Input: part model. Units: mm. Frame: model coordinates. Face numbers are marked on the shaded views. A direction names the side the tool comes from. Coordinates: 2 decimals unless noted, no trailing zeros. Order: outer loops, then holes, each group sorted by start corner. A loop starts at its lowest first (then second) coordinate and runs counter-clockwise, first axis right, second up. Notation, with made-up numbers: (35.25, 36) -> (43.25, 36) arc R14 cw to (43.25, 61) -> close; hole circle Ø2 at (86.5, -27). An arc over 180 degrees is marked (long way). One line per question, with ' | ' between items.
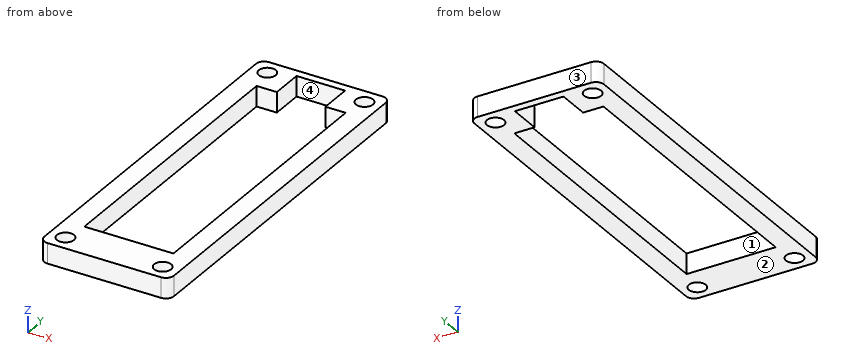
```python
from build123d import *

# Parameters (mm, degrees)
SKETCH_W      = 32
SKETCH_H      = 90
SKETCH_R      = 2.1
EXTRUDE_DEPTH = 5
FILLET_R      = 2


with BuildPart() as part:
    # Sketch → Extrude (new body)
    with BuildSketch(Plane.XY):
        Rectangle(SKETCH_W, SKETCH_H)
        with Locations((-12, 41)):
            Circle(SKETCH_R, mode=Mode.SUBTRACT)
        with Locations((12, 41)):
            Circle(SKETCH_R, mode=Mode.SUBTRACT)
        with Locations((-12, -41)):
            Circle(SKETCH_R, mode=Mode.SUBTRACT)
        with Locations((12, -41)):
            Circle(SKETCH_R, mode=Mode.SUBTRACT)
        Polygon((11, 35), (11, -35), (-11, -35), (-11, 35), (-6, 35), (-6, 43), (6, 43), (6, 35), align=None, mode=Mode.SUBTRACT)
    extrude(amount=EXTRUDE_DEPTH)

    # Fillet
    fillet_edges = [part.edges().sort_by_distance(p)[0] for p in [
        (-16, 45, 2.5),
        (16, 45, 2.5),
        (16, -45, 2.5),
        (-16, -45, 2.5),
    ]]
    fillet(fillet_edges, radius=FILLET_R)


solid = part.part
```
1. Cut plane B-B, the plane x = -5. Return loops of the section in (y, z), and give its area (3 significant figures).
Recorded:
outline: (-45, 0) -> (-35, 0) -> (-35, 5) -> (-45, 5) -> close; (43, 0) -> (45, 0) -> (45, 5) -> (43, 5) -> close | area: 60.0 mm^2
2. Access query for the marked faces 3 and 4. Directions: +Z, -Z, +X, -X, +Y, -Y. A direction counts if a zero-diameter tool reaches every point of the face in a straight line with its end or side. Return the directions, or none.
Recorded:
face 3: +Z, -Z, +X, -X, +Y | face 4: +Z, -Z
3. Mould query, pull axis X, two halves, no side actions, for the marked faces 1 and 2. Classes: released by +X, released by -X, zero draft, split by the parting line, or undercut.
Recorded:
face 1: undercut | face 2: zero draft
4. Cut plane A-A, the plane y = -41. Return loops of the section in (x, z).
Recorded:
outline: (-16, 0) -> (-14.1, 0) -> (-14.1, 5) -> (-16, 5) -> close; (-9.9, 0) -> (9.9, 0) -> (9.9, 5) -> (-9.9, 5) -> close; (14.1, 0) -> (16, 0) -> (16, 5) -> (14.1, 5) -> close
5. Pin query (flat end, axial travel): pin 1 Ø4 at (x, y) = (-12, 41) entering from +Z. Return the tip coordinate at first contact, or that it passes through.
Recorded:
pin 1: passes through
6. Ray query, line 1 (Y direction, x = -12, z = 3.55); line 2 (X direction, y = 0, z = 1.6); line 3 (Y direction, x = -8.5, z = 1.7). Return the intervals inside material, ascending. Write a range as [from, to].
Recorded:
line 1: y = [-45, -43.1], [-38.9, 38.9], [43.1, 45] | line 2: x = [-16, -11], [11, 16] | line 3: y = [-45, -35], [35, 45]
7. Cut plane D-D, the plane z = 3.85. Return loops of the section in (x, y), and give its area (3 significant figures).
Recorded:
outline: (-16, -43) arc R2 ccw to (-14, -45) -> (14, -45) arc R2 ccw to (16, -43) -> (16, 43) arc R2 ccw to (14, 45) -> (-14, 45) arc R2 ccw to (-16, 43) -> close; hole circle Ø4.2 at (-12, -41); hole circle Ø4.2 at (-12, 41); hole (-11, -35) -> (11, -35) -> (11, 35) -> (6, 35) -> (6, 43) -> (-6, 43) -> (-6, 35) -> (-11, 35) -> close; hole circle Ø4.2 at (12, -41); hole circle Ø4.2 at (12, 41) | area: 1,190 mm^2
8. Cut plane C-C, the plane y = -12.5. Return loops of the section in (x, z).
Recorded:
outline: (-16, 0) -> (-11, 0) -> (-11, 5) -> (-16, 5) -> close; (11, 0) -> (16, 0) -> (16, 5) -> (11, 5) -> close
